Input: part model. Units: mm. Frame: model coordinates. A direction names the side the tool comes from. Coordinates: 2 decimals unless noted, no trailing zeros. Loops run counter-clockwise (first coordinate to the right, second up) from the corner with the lowest first, then second, coordinate; pieces in that order, holes last. Notation, with made-up numbers: (-38, 38.5) - (-22, 38.5) arc R17 ccw to (-22, 61.5) - close; hole circle Ø8 at (18.25, -33). An arc over 180 degrees is marked (long way). Use a Markdown table: item, result. Add a question column.
1. Ray query, L1, parallel to X at y = 17.5, z = 5.5 (1 decimal); L2, parallel to X at y = 15.5, z = 5.5 (3 decimals); L3, parallel to Z at x = 34, y = 19.75 (3 decimals). Return the intervals inside material, ascending. Write a range as [from, to].
2. Section query D-D on y = 7.75. Return the cut outline in (x, z) (3 decimals), then the cut area to 3 significant figures.
3. Section query A-A on z = 1. Return the cut outline in (x, y) (3 decimals), then the cut area to 3 significant figures.
4. Section query C-C on x = 31. Return the cut outline in (y, z) (3 decimals), then the cut area to 3 significant figures.
5. Section query B-B on y = 13.5. Return the cut outline in (x, z) (3 decimals).
6. Contact query for flat-ended pins moving along their axis: P1, Ø5, axis at x = 31.5, y = 7, coming from the +Z side (3 decimals); P2, Ø1, axis at y = 18.5, z = 4.5, coming from the +X side; P3, Ø1, axis at y = 16, z = 3.5, coming from the -X side. Output: stop coordinate, or through.
7. Access query for faces 1 (the face through (34.925, 13, 5)), 2 (the face through (7.64, 18.16, 3.13)). Directions: +Z, -Z, +X, -X, +Y, -Y. A direction counts if a zero-diameter tool reaches every point of the face in a straight line with its end or side. Return the directions, or none.
```python
from build123d import *

# Parameters (mm, degrees)
F0_W     = 6.35
F0_H     = 25.4
F1_DEPTH = 6.35
F3_DEPTH = 3.175


with BuildPart() as f1:
    # F0 (on Top) → F1 (new body)
    with BuildSketch(Plane.XY):
        with BuildLine():
            Line((34.925, 25.400001), (34.925, 1e-06))
            Line((34.925, 1e-06), (63.5, 2e-06))
            ThreePointArc((63.5, 2e-06), (56.060512, 17.960514), (38.1, 25.400001))
            Line((38.1, 25.400001), (34.925, 25.400001))
        make_face()
        with BuildLine():
            ThreePointArc((25.4, 25.400001), (7.439487, 17.960513), (0, 0))
            Line((0, 0), (28.575, 1e-06))
            Line((28.575, 1e-06), (28.575, 25.400001))
            Line((28.575, 25.400001), (25.4, 25.400001))
        make_face()
        with Locations((31.75, 12.700001)):
            Rectangle(F0_W, F0_H)
    extrude(amount=F1_DEPTH)

    # F2 (on face) → F3 (cut)
    with BuildSketch(Plane.XY.offset(6.35)):
        Polygon((28.574999, 25.400001), (28.575, 1e-06), (34.925, 1e-06), (34.924999, 25.400001), align=None)
    extrude(amount=-F3_DEPTH, mode=Mode.SUBTRACT)


solid = f1.part
```
Resolved:
| question | item | result |
|---|---|---|
| 1 | L1 | [7, 28.6], [34.9, 56.5] |
| 1 | L2 | [5.278, 28.575], [34.925, 58.222] |
| 1 | L3 | [0, 3.175] |
| 2 | outline | (1.211, 0) - (62.289, 0) - (62.289, 6.35) - (34.925, 6.35) - (34.925, 3.175) - (28.575, 3.175) - (28.575, 6.35) - (1.211, 6.35) - close |
| 2 | area | 368 mm² |
| 3 | outline | (0, 0) - (63.5, 0) arc R25.4 ccw to (38.1, 25.4) - (25.4, 25.4) arc R25.4 ccw to start |
| 3 | area | 1,340 mm² |
| 4 | outline | (0, 0) - (25.4, 0) - (25.4, 3.175) - (0, 3.175) - close |
| 4 | area | 80.6 mm² |
| 5 | outline | (3.885, 0) - (59.615, 0) - (59.615, 6.35) - (34.925, 6.35) - (34.925, 3.175) - (28.575, 3.175) - (28.575, 6.35) - (3.885, 6.35) - close |
| 6 | P1 | z = 3.175 |
| 6 | P2 | x = 56.02 |
| 6 | P3 | x = 5.28 |
| 7 | face 1 | +Z, +Y, -Y |
| 7 | face 2 | +Z, -Z, -X, +Y |
